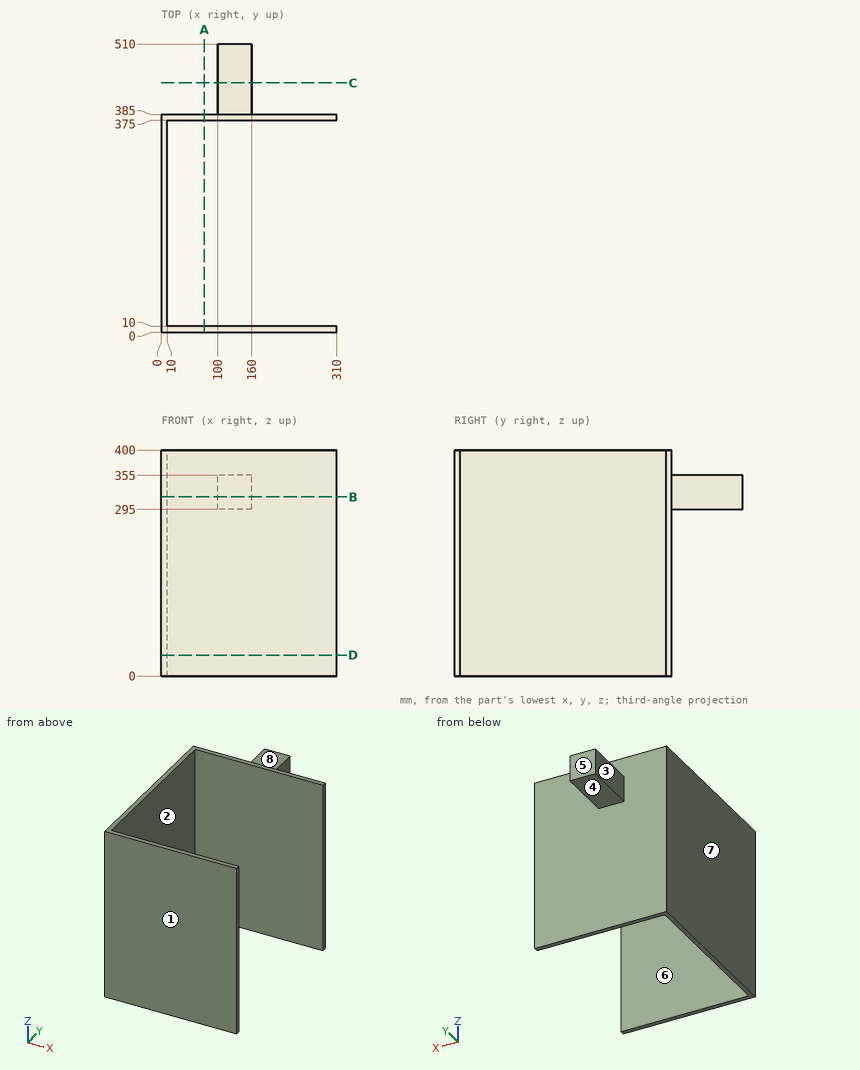
Verification items for this drawing (mm, ordinates from the low corner). A direction names the side the tool comes from. Give positions to 0.01 mm unless a question says otherwise; leave off trailing zeros. Loops run counter-clockwise (first coordinate to the right, second up) from the corner with the lowest first, then second, coordinate; pieces in that order, holes last. Notation, with made-up numbers: M -1,2 L 53,2 A24 ccw 53,15 Z; hole C 49.25,4.5 d5. An arc over 180 degrees is marked long. Answer in a Markdown table with one row per item.
1) Depth check by flat-ended pin: pin 1 (3 mm diameter, centred on x = 236, z = 59, fed in from -Y); pin 2 (3 mm diameter, centred on x = 157.5, z = 233.5, fed in from +Y); pin 3 (18 mm diameter, centred on x = 120, y = 452, fed in from -Z). Enter the tip coordinate at first touch or a pass-through.
Solutions:
| item | result |
|---|---|
| pin 1 | stops at y = 0 |
| pin 2 | stops at y = 385 |
| pin 3 | stops at z = 295 |
2) Thickness scan on line 1 (Y direction, x = 249.5, z = 67.5); line 2 (X direction, y = 162, z = 210). Record the ranges inside material, lowest first.
Solutions:
| item | result |
|---|---|
| line 1 | y = 0 to 10, 375 to 385 |
| line 2 | x = 0 to 10 |
3) Mould release check, pull along Y, two halves, no side actions. Record for the marked faces 1, 2 and 3: released by +Y, released by -Y, zero draft, split by the parting line, or undercut.
Solutions:
| item | result |
|---|---|
| face 1 | released by -Y |
| face 2 | undercut |
| face 3 | zero draft |
4) Cross-section at B-B (z = 317). Enter the section's corners in (x, y).
Solutions:
| item | result |
|---|---|
| outline | M 0,0 L 310,0 L 310,10 L 10,10 L 10,375 L 310,375 L 310,385 L 160,385 L 160,510 L 100,510 L 100,385 L 0,385 Z |
5) Tool access check on the marked faces 4, 5, 6, 7 and 8. Record the directions out of +Z, -Z, +X, -X, +Y, -Y that give a thin tool (end or side, any length) a straight path to the whole face; none if there is none.
Solutions:
| item | result |
|---|---|
| face 4 | -Z, +X, -X, +Y |
| face 5 | +Z, -Z, +X, -X, +Y |
| face 6 | +Z, -Z, +X |
| face 7 | +Z, -Z, -X, +Y, -Y |
| face 8 | +Z, +X, -X, +Y |
6) Cross-section at A-A (x = 76). Enter the section's corners in (y, z), plus the area to 3 significant figures.
Solutions:
| item | result |
|---|---|
| outline | M 0,0 L 10,0 L 10,400 L 0,400 Z; M 375,0 L 385,0 L 385,400 L 375,400 Z |
| area | 8,000 mm^2 |
7) Cross-section at C-C (y = 441). Enter the section's corners in (x, z).
Solutions:
| item | result |
|---|---|
| outline | M 100,295 L 160,295 L 160,355 L 100,355 Z |
8) Cross-section at D-D (z = 37). Enter the section's corners in (x, y), plus the area to 3 significant figures.
Solutions:
| item | result |
|---|---|
| outline | M 0,0 L 310,0 L 310,10 L 10,10 L 10,375 L 310,375 L 310,385 L 0,385 Z |
| area | 9,850 mm^2 |
